```python
from build123d import *

# Parameters (mm, degrees)
SKETCH1_R               = 20
BOSS_EXTRUDE1_DEPTH     = 50
SKETCH3_R               = 40
BOSS_EXTRUDE2_DEPTH     = 5
CHAMFER1_SIZE           = 2
CUT_EXTRUDE1_DEPTH      = 120.268604419
CUT_EXTRUDE1_DEPTH_BACK = 120.268604419
SKETCH4_R               = 2.5
FILLET1_R               = 3


with BuildPart() as part:
    # Sketch1 → Boss-Extrude1 (new, symmetric)
    with BuildSketch(Plane(origin=(0, 0, 0), x_dir=(1, 0, 0), z_dir=(0, 1, 0))):
        with Locations(Location((0, 0, 0), (0, 0, 270))):
            Circle(SKETCH1_R)
    extrude(amount=BOSS_EXTRUDE1_DEPTH, both=True)

    # Sketch3 → Boss-Extrude2 (add)
    with BuildSketch(Plane(origin=(0, 50, 0), x_dir=(1, 0, 0), z_dir=(0, 1, 0))):
        with Locations(Location((0, 0, 0), (0, 0, 270))):
            Circle(SKETCH3_R)
    extrude(amount=BOSS_EXTRUDE2_DEPTH)

    # Chamfer1
    chamfer1_edges = [part.edges().sort_by_distance(p)[0] for p in [
        (0, 55, -40),
    ]]
    chamfer(chamfer1_edges, length=CHAMFER1_SIZE)

    # Sketch4 → Cut-Extrude1 (cut, two sides: drawn at the far end of the back side and taken through both)
    with BuildSketch(Plane(origin=(0, 55, 0), x_dir=(1, 0, 0), z_dir=(0, 1, 0)).offset(-CUT_EXTRUDE1_DEPTH_BACK)):
        with Locations(Location((0, 30, 0), (0, 0, 270))):
            Circle(SKETCH4_R)
    extrude(amount=CUT_EXTRUDE1_DEPTH + CUT_EXTRUDE1_DEPTH_BACK, mode=Mode.SUBTRACT)

    # Fillet1
    fillet1_edges = [part.edges().sort_by_distance(p)[0] for p in [
        (0, 50, -40),
    ]]
    fillet(fillet1_edges, radius=FILLET1_R - 0.0001)  # a hair under: the kernel refuses the full size


solid = part.part
```
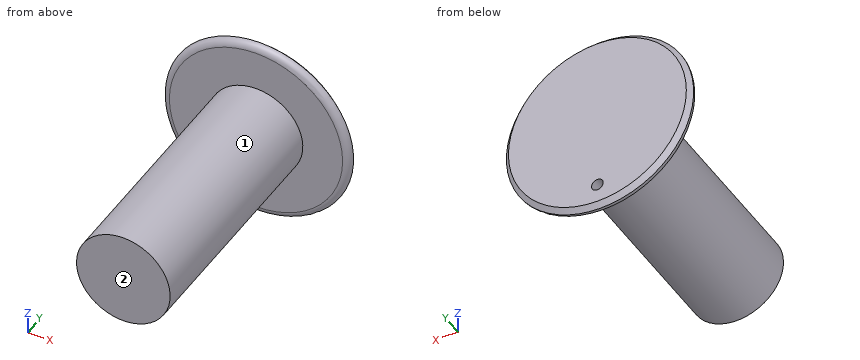
Verification items for the finished model (mm, model axes). Face numbers are marked on the shaded views. A direction names the side the tool comes from. Coordinates: 2 decimals unless noted, no trailing zeros. Loops run counter-clockwise (first coordinate to the right, second up) from the corner with the lowest first, then second, coordinate; pieces in that order, holes last. Notation, with made-up numbers: (9.25, 28) -> (55.25, 28) arc R13 cw to (55.25, 41) -> close; hole circle Ø11 at (18.5, 68). An arc over 180 degrees is marked (long way). Answer in a Markdown table with one row per item. Add a question column.
1. Section check C-C, the plane y = 11. Enter the section's corners in (x, z), then the cut area to 3 significant figures.
2. Depth check by flat-ended pin: P1, Ø3, axis at y = 10.5, z = -10, coming from the -X side; P2, Ø4, axis at x = -15.5, y = 5.5, coming from the -Z side; P3, Ø8, axis at x = 0, z = -30, coming from the +Y side; P4, Ø4, axis at x = -4, y = -29.5, coming from the +Z side. Enter the tip coordinate at first touch or a pass-through.
3. Material ranges on probe 1 along X at (y, z) = (53, -30); probe 2 along X at (y, z) = (51, -30); probe 3 along Z at (x, y) = (0, 53.15), recorded low to high. Write a range as [from, to].
4. Access from +Z, -Z, +X, -X, +Y, -Y to the whole of each face (thin tool, end or side, straight path). Record for the marked faces 1 and 2.
Derived:
| question | item | result |
|---|---|---|
| 1 | outline | circle Ø40 at (0, 0) |
| 1 | area | 1,260 mm² |
| 2 | P1 | stops at x = -18.1 |
| 2 | P2 | stops at z = -14.76 |
| 2 | P3 | stops at y = 55 |
| 2 | P4 | stops at z = 19.9 |
| 3 | probe 1 | x = [-26.46, -2.5], [2.5, 26.46] |
| 3 | probe 2 | x = [-25.29, -2.5], [2.5, 25.29] |
| 3 | probe 3 | z = [-39.85, -32.5], [-27.5, 39.85] |
| 4 | face 1 | -Y |
| 4 | face 2 | +Z, -Z, +X, -X, -Y |
